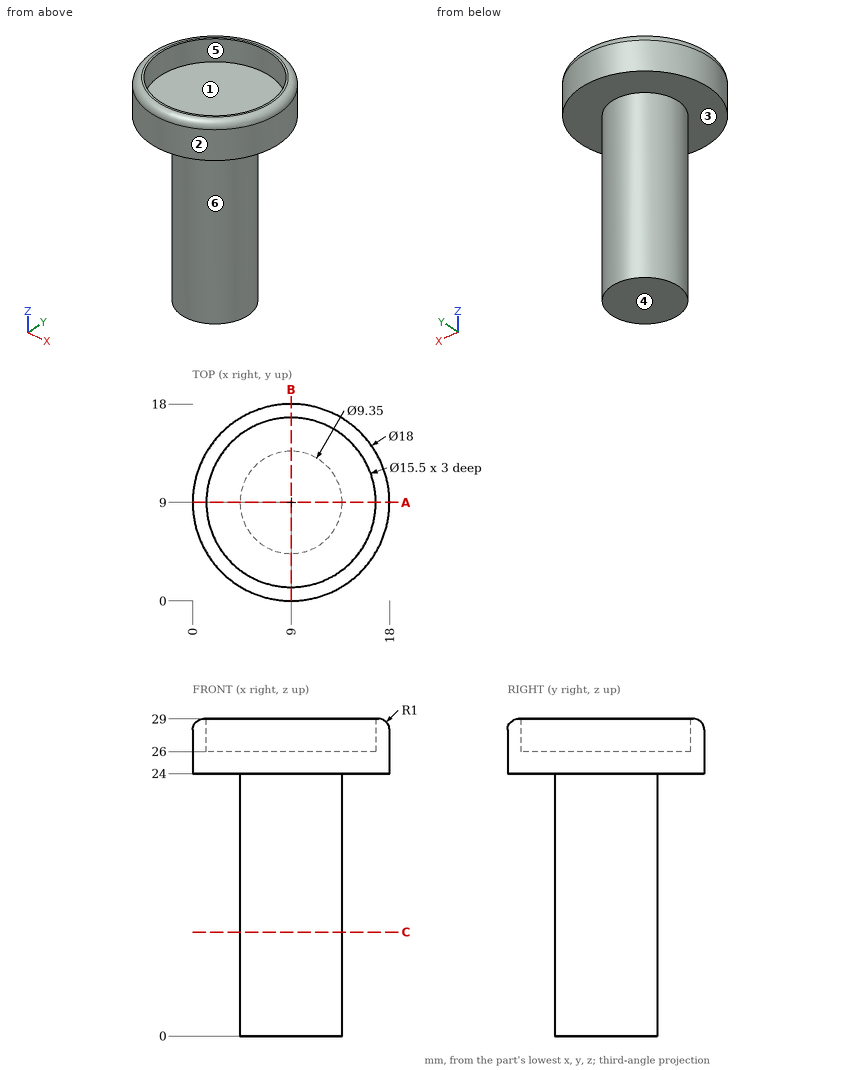
For this review, use the dimensioned drawing (mm, ordinates from the lowest corner) and the shaded views. A direction names the side the tool comes from. Coordinates: 2 decimals unless noted, no trailing zeros. Order: outer loops, then holes, each group sorted by start corner. A loop starts at its lowest first (then second) coordinate and runs counter-clockwise, first axis right, second up. Notation, with made-up numbers: M 66.5,38 L 85.5,38 A19 cw 85.5,63 Z; hole C 83.25,27.25 d9. An arc over 180 degrees is marked long. Answer as a JSON object with one key per item and string values. Group by question number.
1) Add section A-A, the plane y = 9. Write out the cut boundary in (x, z) (3 decimals), then the cut area to 3 significant figures.
2) Add section C-C, the plane z = 9.5. Write out the cut boundary in (x, y) (3 decimals), then the cut area to 3 significant figures.
3) For pin 1 (10 mm diameter, centred on y = 7.5, z = 4, fed in from +X) (3 decimals); pin 2 (1 mm diameter, centred on x = 14.5, y = 11.5, fed in from +Z); pin 3 (1.5 mm diameter, centred on x = 12, z = 13, fed in from +Y); pin 4 (1 mm diameter, centred on x = 5, y = 2.5, fed in from +Z), all flat-tipped, find the tip position at first contact; note any pin that passes through.
4) Wall thickness on L1, parallel to Y at x = 9, z = 27.95; L2, parallel to Z at x = 5.5, y = 6.75; L3, parallel to Z at x = 2, y = 6.5: over which ranges is each line inside the solid? List them lowest first.
5) Tool access review of the marked faces 1, 2 and 3: name each direction out of +Z, -Z, +X, -X, +Y, -Y from which nothing blocks a thin tool from reaching the whole face with its end or side.
6) Mouldability with a two-part tool opening along Y and no side actions: class the marked faces 4, 5 and 6 as pulls with the +Y half, pulls with the -Y half, needs draft (parallel to the pull), parting line crosses it, or undercut.
Computed values:
{
 "1": {"outline": "M 0,24 L 4.325,24 L 4.325,0 L 13.675,0 L 13.675,24 L 18,24 L 18,28 A1 ccw 17,29 L 16.75,29 L 16.75,26 L 1.25,26 L 1.25,29 L 1,29 A1 ccw 0,28 Z", "area": "267 mm^2"},
 "2": {"outline": "C 9,9 d9.35", "area": "68.7 mm^2"},
 "3": {"pin 1": "stops at x = 13.675", "pin 2": "stops at z = 26", "pin 3": "stops at y = 13.1", "pin 4": "stops at z = 29"},
 "4": {"L1": "y = 0 to 1.25, 16.75 to 18", "L2": "z = 0 to 26", "L3": "z = 24 to 26"},
 "5": {"face 1": "+Z", "face 2": "+Z, -Z", "face 3": "-Z"},
 "6": {"face 4": "needs draft", "face 5": "undercut", "face 6": "parting line crosses it"}
}
